Source: CAD feature listing. Evaluate the final solid. Frame: model axes, mm. Face numbers are marked on the shaded views. A direction names the side the tool comes from. Coordinates: 2 decimals unless noted, no trailing zeros. Loops run counter-clockwise (first coordinate to the right, second up) from the corner with the lowest first, then second, coordinate; pieces in that order, holes last. Notation, with made-up numbers: (6, -28.75) -> (61, -28.75) arc R20 ccw to (61, -10.75) -> close; hole circle Ø5 at (-34, 79). An arc over 180 degrees is marked (long way). Answer as CSV lines item,"result".
from build123d import *

# Parameters (mm, degrees)
BOSS_EXTRUDE1_DEPTH      = 18.15
BOSS_EXTRUDE1_DEPTH_BACK = 1
SKETCH1_W                = 78.86
SKETCH1_H                = 48
SHELL1_T                 = -2
BOSS_EXTRUDE2_START      = 3
SKETCH4_R                = 2
BOSS_EXTRUDE2_DEPTH      = 4.4
CHAMFER2_SIZE            = 3.4
CHAMFER3_SIZE            = 3.4
CHAMFER4_SIZE            = 3.4
BOSS_EXTRUDE4_DEPTH      = 17.15
CUT_EXTRUDE4_DEPTH       = 60.613659429
CUT_EXTRUDE4_DEPTH_BACK  = 22
SKETCH14_R               = 1.6
FILLET1_R                = 2
CUT_EXTRUDE9_REACH       = 86.549
SKETCH17_W               = 12.51
SKETCH17_H               = 7.45
SKETCH21_R               = 1.6
CUT_EXTRUDE10_DEPTH      = 4.2


with BuildPart() as part:
    # Sketch1 → Boss-Extrude1 (new, two sides: drawn at the far end of the back side and taken through both)
    with BuildSketch(Plane(origin=(0, 0, 0), x_dir=(1, 0, 0), z_dir=(0, 1, 0)).offset(-BOSS_EXTRUDE1_DEPTH_BACK)):
        with Locations((-11.43075, -0.5)):
            Rectangle(SKETCH1_W, SKETCH1_H)
    extrude(amount=BOSS_EXTRUDE1_DEPTH + BOSS_EXTRUDE1_DEPTH_BACK)

    # Shell1
    shell1_openings = [part.faces().sort_by_distance(p)[0] for p in [
        (-11.43075, 18.15, 0.5),
    ]]
    offset(amount=SHELL1_T, openings=shell1_openings, kind=Kind.INTERSECTION)

    # Sketch4 → Boss-Extrude2 (add)
    with BuildSketch(Plane(origin=(0, 1, 0), x_dir=(1, 0, 0), z_dir=(0, 1, 0)).offset(BOSS_EXTRUDE2_START)):
        with Locations(Location((-35.69075, -17.71, 0), (0, 0, 270))):
            Circle(SKETCH4_R)
        with Locations(Location((-4.71075, -11.75, 0), (0, 0, 270))):
            Circle(SKETCH4_R)
        with Locations(Location((11.67925, 17.1, 0), (0, 0, 270))):
            Circle(SKETCH4_R)
    extrude(amount=-BOSS_EXTRUDE2_DEPTH)

    # Chamfer2
    # the kernel refuses this chamfer: 3.4 mm, written as the material it adds along each edge
    with BuildSketch(Plane(origin=(-4.71075, 1, 11.75), x_dir=(0, 0, 1), z_dir=(-1, 0, 0))) as chamfer2_piece_1_section:
        Polygon((2 + CHAMFER2_SIZE, 0), (2, CHAMFER2_SIZE), (2, 0), align=None)
    chamfer2_piece_1 = revolve(axis=Axis((-4.71075, 1, 11.75), (0, 1, 0)), mode=Mode.PRIVATE)
    chamfer2_piece_1 = split(chamfer2_piece_1, bisect_by=Plane(origin=(-4.71075, 4, 7.837068743), z_dir=(0, -1, 0)), keep=Keep.TOP, mode=Mode.PRIVATE)
    add(chamfer2_piece_1)

    # Chamfer3
    # the kernel refuses this chamfer: 3.4 mm, written as the material it adds along each edge
    with BuildSketch(Plane(origin=(11.67925, 1, -17.1), x_dir=(0, 0, 1), z_dir=(-1, 0, 0))) as chamfer3_piece_1_section:
        Polygon((2 + CHAMFER3_SIZE, 0), (2, CHAMFER3_SIZE), (2, 0), align=None)
    chamfer3_piece_1 = revolve(axis=Axis((11.67925, 1, -17.1), (0, 1, 0)), mode=Mode.PRIVATE)
    chamfer3_piece_1 = split(chamfer3_piece_1, bisect_by=Plane(origin=(11.67925, 4, -21.012931257), z_dir=(0, -1, 0)), keep=Keep.TOP, mode=Mode.PRIVATE)
    add(chamfer3_piece_1)

    # Chamfer4
    # the kernel refuses this chamfer: 3.4 mm, written as the material it adds along each edge
    with BuildSketch(Plane(origin=(-35.69075, 1, 17.71), x_dir=(0, 0, 1), z_dir=(-1, 0, 0))) as chamfer4_piece_1_section:
        Polygon((2 + CHAMFER4_SIZE, 0), (2, CHAMFER4_SIZE), (2, 0), align=None)
    chamfer4_piece_1 = revolve(axis=Axis((-35.69075, 1, 17.71), (0, 1, 0)), mode=Mode.PRIVATE)
    chamfer4_piece_1 = split(chamfer4_piece_1, bisect_by=Plane(origin=(-35.69075, 4, 13.797068743), z_dir=(0, -1, 0)), keep=Keep.TOP, mode=Mode.PRIVATE)
    add(chamfer4_piece_1)

    # Sketch9 → Boss-Extrude4 (add)
    with BuildSketch(Plane(origin=(0, 1, 0), x_dir=(1, 0, 0), z_dir=(0, 1, 0))):
        Polygon((-48.86075, 16.53575), (-43.8965, 21.5), (-48.86075, 21.5), align=None)
        Polygon((21.035, 21.5), (25.99925, 16.53575), (25.99925, 21.5), align=None)
        Polygon((25.99925, -17.53575), (21.035, -22.5), (25.99925, -22.5), align=None)
        Polygon((-43.8965, -22.5), (-48.86075, -17.53575), (-48.86075, -22.5), align=None)
    extrude(amount=BOSS_EXTRUDE4_DEPTH)

    # Sketch14 → Cut-Extrude4 (cut, two sides: drawn at the far end of the back side and taken through both)
    with BuildSketch(Plane(origin=(0, 18.15, 0), x_dir=(1, 0, 0), z_dir=(0, 1, 0)).offset(-CUT_EXTRUDE4_DEPTH_BACK)):
        with Locations(Location((-48.36075, 21, 0), (0, 0, 90))):
            Circle(SKETCH14_R)
        with Locations(Location((25.49925, 21, 0), (0, 0, 90))):
            Circle(SKETCH14_R)
        with Locations(Location((25.49925, -21.75, 0), (0, 0, 90))):
            Circle(SKETCH14_R)
        with Locations(Location((-48.36075, -21.75, 0), (0, 0, 90))):
            Circle(SKETCH14_R)
    extrude(amount=CUT_EXTRUDE4_DEPTH + CUT_EXTRUDE4_DEPTH_BACK, mode=Mode.SUBTRACT)

    # Fillet1
    fillet1_edges = [part.edges().sort_by_distance(p)[0] for p in [
        (-50.86075, 8.575, -23.5),
        (27.99925, 8.575, -23.5),
        (27.99925, 8.575, 24.5),
        (-50.86075, 8.575, 24.5),
    ]]
    fillet(fillet1_edges, radius=FILLET1_R)

    # Sketch17 → Cut-Extrude9 (cut, up to next)
    with BuildSketch(Plane(origin=(27.99925, 0, 0), x_dir=(0, 0, -1), z_dir=(1, 0, 0)), mode=Mode.PRIVATE) as cut_extrude9_sk1:
        with Locations((10.785, 6.425)):
            Rectangle(SKETCH17_W, SKETCH17_H)
    cut_extrude9_tool1 = extrude(cut_extrude9_sk1.sketch, amount=-CUT_EXTRUDE9_REACH, mode=Mode.PRIVATE) & part.part
    add(cut_extrude9_tool1.solids().sort_by_distance((27.99925, 6.425, -10.785))[0], mode=Mode.SUBTRACT)

    # Sketch21 → Cut-Extrude10 (cut)
    with BuildSketch(Plane(origin=(0, 4, 0), x_dir=(1, 0, 0), z_dir=(0, 1, 0))):
        with Locations(Location((11.67925, 17.1, 0), (0, 0, 270))):
            Circle(SKETCH21_R)
        with Locations(Location((-4.71075, -11.75, 0), (0, 0, 270))):
            Circle(SKETCH21_R)
        with Locations(Location((-35.69075, -17.71, 0), (0, 0, 270))):
            Circle(SKETCH21_R)
    extrude(amount=-CUT_EXTRUDE10_DEPTH, mode=Mode.SUBTRACT)


solid = part.part
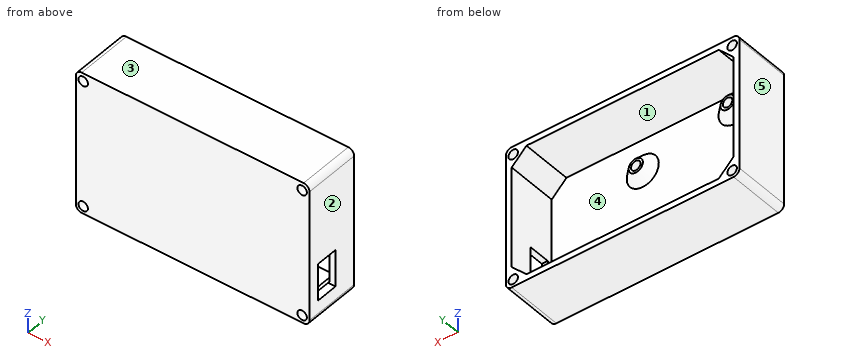
(1) Access query for the marked faces 1 and 2. Directions: +Z, -Z, +X, -X, +Y, -Y. A direction counts if a zero-diameter tool reaches every point of the face in a straight line with its end or side. Return the directions, or none.
Computed values:
face 1,"+Y"
face 2,"+Z, -Z, +X, +Y, -Y"
(2) Cut plane D-D (x = -16). Return the cut outline in (y, z), then the cut area to 3 significant figures.
Computed values:
outline,"(-1, -23.5) -> (18.15, -23.5) -> (18.15, -21.5) -> (1, -21.5) -> (1, 22.5) -> (18.15, 22.5) -> (18.15, 24.5) -> (-1, 24.5) -> close"
area,"165 mm^2"
(3) Draft query along Z for the marked faces 3, 4 and 5. Return one class per face: released by +Z, released by -Z, zero draft, split by the parting line, or undercut.
Computed values:
face 3,"released by +Z"
face 4,"undercut"
face 5,"zero draft"
(4) Pin query (flat end, axial travel): pin 1 Ø3.5 at (x, z) = (-48.36, -21) entering from -Y; pin 2 Ø5.5 at (x, z) = (11.5, -17.5) entering from +Y; pin 3 Ø3 at (x, z) = (-8.5, 2) entering from +Y; pin 4 Ø1.4 at (x, z) = (-5.5, 11.5) entering from +Y. Return the tip coordinate at first contact, or that it passes through.
Computed values:
pin 1,"y = -1"
pin 2,"y = 4"
pin 3,"y = 1"
pin 4,"y = -0.2"
(5) Cut plane A-A (y = 5.5). State how many separate pieces and enclosed holes the cut face has, then the cut area to 3 significant figures.
Computed values:
separate pieces,"1"
enclosed holes,"4"
area,"480 mm^2"
(6) Material intervals for L1, parallel to Z at x = -12, y = 10; L2, parallel to Z at x = -34.5, y = 3.5; L3, parallel to X at y = 6.25, z = -2, sorted ascending. Write a range as [from, to].
Computed values:
L1,"[-23.5, -21.5], [22.5, 24.5]"
L2,"[-23.5, -21.5], [15.07, 16.64], [18.78, 20.35], [22.5, 24.5]"
L3,"[-50.86, -48.86], [26, 28]"
(7) Cut plane B-B (z = -1). Return the cut outline in (x, y), then the cut area to 3 significant figures.
Computed values:
outline,"(-50.86, -1) -> (28, -1) -> (28, 18.15) -> (26, 18.15) -> (26, 1) -> (-48.86, 1) -> (-48.86, 18.15) -> (-50.86, 18.15) -> close"
area,"226 mm^2"
